CAD build for the part. Positions are in the model's coordinates, mm. A direction names the side the tool comes from. Give positions to 0.01 mm unless a question says otherwise; leave off trailing zeros. Loops run counter-clockwise (first coordinate to the right, second up) from the corner with the lowest first, then second, coordinate; pieces in that order, holes last.
Item 1: Which spindle directions (+Z, -Z, +X, -X, +Y, -Y) get a long thin tool onto all of the face, cutting with end or side? Do faces 4 (the flat face through (-1, 19.05, -8)), 5 (the cylindrical face through (1.38, 11.54, -6.2)). Say none if no direction does.
Item 2: Saw through at C-C on x = 31.75. Give the cut face in (y, z) (3 decimals), plus the area to 3 significant figures.
Item 3: Saw through at B-B on z = 0. Give the cut face in (x, y), plus the area to 3 significant figures.
Item 4: Saw through at D-D on y = 12. Give the number of separate pieces and of enclosed holes in the cut face, plus the area to 3 significant figures.
Item 5: Probe probe 1 along Z at (x, y) = (-31.75, 8) (3 decimals); probe 2 along Z at (x, y) = (0, 1) (3 decimals); probe 3 along X at (y, z) = (14.75, 23). List the from-to ranges inside material, lowest first.
Item 6: Saw through at A-A on x = 0. Give the cut face in (y, z) (3 decimals).
Item 7: Mould opens along Z. For faces 1 (the cylindrical face through (-41.98, 9.63, 14.53)), 2 (the flat face through (-1, 9, -34.925)), 3 (the flat face through (-1, 0, -8)) say: released by +Z, released by -Z, zero draft, split by the parting line, or undercut.
Item 8: Drop a flat-ended pin along its axis: P1, Ø23.5, axis at x = 31.75, z = 15.875, coming from the -Y side (3 decimals). Give the stop position or say it passes through.
from build123d import *

# Parameters (mm, degrees)
SKETCH1_W                                       = 101.6
SKETCH1_H                                       = 69.85
EXTRUDE1_DEPTH                                  = 19.05
F_13_16_0_8125_DIAMETER_HOLE1_AT_2_COUNT        = 2
F_13_16_0_8125_DIAMETER_HOLE1_AT_2_PITCH        = 31.75
F_13_16_0_8125_DIAMETER_HOLE1_AT_3_COUNT        = 2
F_13_16_0_8125_DIAMETER_HOLE1_AT_3_PITCH        = 70.995158286
F_13_16_0_8125_DIAMETER_HOLE1_AT_4_COUNT        = 2
F_13_16_0_8125_DIAMETER_HOLE1_AT_4_PITCH        = 63.5
CBORE_FOR_10_SOCKET_HEAD_CAP_SCREW1_D           = 5.6134
CBORE_FOR_10_SOCKET_HEAD_CAP_SCREW1_CBORE_D     = 12.7
CBORE_FOR_10_SOCKET_HEAD_CAP_SCREW1_CBORE_DEPTH = 15.24
CHAMFER1_SIZE                                   = 0.508


with BuildPart() as part:
    # Sketch1 → Extrude1 (new body)
    with BuildSketch(Plane(origin=(0, 0, 0), x_dir=(1, 0, 0), z_dir=(0, 1, 0))):
        Rectangle(SKETCH1_W, SKETCH1_H)
    extrude(amount=EXTRUDE1_DEPTH)

    # Sketch3 → 13/16 (0.8125) Diameter Hole1 (revolve, cut)
    with BuildSketch(Plane(origin=(31.75, 19.05, 15.875), x_dir=(0, 0, 1), z_dir=(1, 0, 0))):
        Polygon((0, 0), (0, 19.05), (12.065, 19.05), (10.31875, 17.30375), (10.31875, 1.74625), (12.065, 0), align=None)
    f_13_16_0_8125_diameter_hole1 = revolve(axis=Axis((31.75, 25.4, 15.875), (0, -1, 0)), mode=Mode.SUBTRACT)

    # 13/16 (0.8125) Diameter Hole1 at 2: 13/16 (0.8125) Diameter Hole1 ×2
    with Locations(*[(0, 0, -i * F_13_16_0_8125_DIAMETER_HOLE1_AT_2_PITCH) for i in range(1, F_13_16_0_8125_DIAMETER_HOLE1_AT_2_COUNT)]):
        add(f_13_16_0_8125_diameter_hole1, mode=Mode.SUBTRACT)

    # 13/16 (0.8125) Diameter Hole1 at 3: 13/16 (0.8125) Diameter Hole1 ×2
    with Locations(*[Vector(-0.894427191, 0, -0.447213595) * (i * F_13_16_0_8125_DIAMETER_HOLE1_AT_3_PITCH) for i in range(1, F_13_16_0_8125_DIAMETER_HOLE1_AT_3_COUNT)]):
        add(f_13_16_0_8125_diameter_hole1, mode=Mode.SUBTRACT)

    # 13/16 (0.8125) Diameter Hole1 at 4: 13/16 (0.8125) Diameter Hole1 ×2
    with Locations(*[(-i * F_13_16_0_8125_DIAMETER_HOLE1_AT_4_PITCH, 0, 0) for i in range(1, F_13_16_0_8125_DIAMETER_HOLE1_AT_4_COUNT)]):
        add(f_13_16_0_8125_diameter_hole1, mode=Mode.SUBTRACT)

    # CBORE for #10 Socket Head Cap Screw1 (through all)
    with Locations(Plane(origin=(0, 19.05, 0), x_dir=(-1, 0, 0), z_dir=(0, 1, 0))):
        with Locations((0, 0)):
            CounterBoreHole(CBORE_FOR_10_SOCKET_HEAD_CAP_SCREW1_D / 2, CBORE_FOR_10_SOCKET_HEAD_CAP_SCREW1_CBORE_D / 2, CBORE_FOR_10_SOCKET_HEAD_CAP_SCREW1_CBORE_DEPTH)

    # Chamfer1
    chamfer1_edges = [part.edges().sort_by_distance(p)[0] for p in [
        (50.8, 19.05, 0),
        (0, 19.05, -34.925),
        (-50.8, 19.05, 0),
        (0, 0, -34.925),
        (50.8, 0, 0),
        (0, 0, 34.925),
        (-50.8, 0, 0),
        (0, 19.05, 34.925),
        (-50.8, 9.525, -34.925),
        (50.8, 9.525, -34.925),
        (50.8, 9.525, 34.925),
        (-50.8, 9.525, 34.925),
    ]]
    chamfer(chamfer1_edges, length=CHAMFER1_SIZE)


solid = part.part
Results below:
1. face 4: +Z, -Z, +X, -X, +Y
1. face 5: +Y
2. outline: (0, -34.417) - (0.508, -34.925) - (18.542, -34.925) - (19.05, -34.417) - (19.05, -27.94) - (17.304, -26.194) - (1.746, -26.194) - (0, -27.94) - close; (0, -3.81) - (1.746, -5.556) - (17.304, -5.556) - (19.05, -3.81) - (19.05, 3.81) - (17.304, 5.556) - (1.746, 5.556) - (0, 3.81) - close; (0, 27.94) - (1.746, 26.194) - (17.304, 26.194) - (19.05, 27.94) - (19.05, 34.417) - (18.542, 34.925) - (0.508, 34.925) - (0, 34.417) - close
2. area: 532 mm2
3. outline: (-50.8, 0.51) - (-50.29, 0) - (-2.81, 0) - (-2.81, 3.81) - (-6.35, 3.81) - (-6.35, 19.05) - (-50.29, 19.05) - (-50.8, 18.54) - close; (2.81, 0) - (50.29, 0) - (50.8, 0.51) - (50.8, 18.54) - (50.29, 19.05) - (6.35, 19.05) - (6.35, 3.81) - (2.81, 3.81) - close
3. area: 1,720 mm2
4. separate pieces: 1
4. enclosed holes: 5
4. area: 5,630 mm2
5. probe 1: z = -34.925 to -26.194, -5.556 to 5.556, 26.194 to 34.925
5. probe 2: z = -34.925 to -2.807, 2.807 to 34.925
5. probe 3: x = -50.8 to -39.21, -24.29 to 24.29, 39.21 to 50.8
6. outline: (0, -34.417) - (0.508, -34.925) - (18.542, -34.925) - (19.05, -34.417) - (19.05, -6.35) - (3.81, -6.35) - (3.81, -2.807) - (0, -2.807) - close; (0, 2.807) - (3.81, 2.807) - (3.81, 6.35) - (19.05, 6.35) - (19.05, 34.417) - (18.542, 34.925) - (0.508, 34.925) - (0, 34.417) - close
7. face 1: undercut
7. face 2: released by -Z
7. face 3: zero draft
8. P1: stops at y = 0.315
